The listing builds one solid part. Answer for the finished solid, in the listing's coordinates (mm). A direction names the side the tool comes from. Round coordinates to 2 decimals unless told otherwise and drop trailing zeros. Write each loop counter-clockwise with the first axis right and the second up, starting at its lowest first coordinate (ties: lowest second). Pieces come first, ordered by that corner, then holes. Notation, with made-up numbers: (-10.5, 21.5) - (-6.5, 21.5) arc R19 cw to (-6.5, 36.5) - close; hole circle Ø1 at (10, 88.25). An arc over 180 degrees is marked (long way). Answer as CSV lines item,"result". Start each with the question number.
Item 1: A cutting plane is placed at B-B on x = 0. Determine the outline of the cut face in (y, z), and give its area (3 significant figures).
Item 2: Straight lines are drawn through the part: line 1 along Z through (x, y) = (-1.5, 2.25); line 2 along Z through (x, y) = (-1.25, 5.25); line 3 along Y through (x, z) = (-2.25, 1.5). For each, find the intervals that lie inside material, in ascending order. Write a range as [from, to].
Item 3: Which of the six approach directions +Z, -Z, +X, -X, +Y, -Y give full straight-line access (tool end or side, diameter ignored) to faces 1 (the cylindrical face through (-0.54, 1.48, -2.44)), 2 (the flat face through (0, 0, 0))?
Item 4: Flat-ended cylindrical pins translate along their axes: pin 1 (4 mm diameter, centred on y = 1.5, z = -1.5, fed in from -X); pin 2 (3 mm diameter, centred on x = -2, y = 2.5, fed in from +Z); pin 3 (2 mm diameter, centred on y = 5.5, z = -0.5, fed in from -X). Find the tip coordinate at first contact, or state that the pin passes through.
Item 5: A cutting plane is placed at C-C on y = 2.75. Determine the outline of the cut face in (x, z), and give its area (3 significant figures).
Item 6: A cutting plane is placed at A-A on z = 0. Determine the outline of the cut face in (x, y), and give its area (3 significant figures).
Item 7: A cutting plane is placed at D-D on y = 3.5. Determine the outline of the cut face in (x, z).
Autodesk Inventor part; units mm, degrees
ref_plane "YZ Plane" through (0, 0, 0) normal (1, 0, 0) x (0, 1, 0)
ref_plane "XZ Plane" through (0, 0, 0) normal (0, 1, 0) x (-1, 0, 0)
ref_plane "XY Plane" through (0, 0, 0) normal (0, 0, 1) x (1, 0, 0)
sketch "Szkic1" plane through (0, 0, 0) normal (0, 1, 0) x (-1, 0, 0)
  circle A0 centre (0, 0) radius 4
  dimension "d0" = 8
extrude "Wyciągnięcie proste1" add sketch "Szkic1" along normal blind 7
fillet "Zaokrąglenie1" radius 4 1 edges at (4, 7, 0)
sketch "Szkic2" plane through (0, 0, 0) normal (0, -1, 0) x (1, 0, 0)
  circle A0 centre (0, 0) radius 2.5
  circle A1 centre (0, 0) radius 4
  dimension "d4" = 5
  dimension "d5" = 8
extrude "Wyciągnięcie proste2" cut sketch "Szkic2" against normal blind 3
properties part number "GumoweTrzymadlo" material "Tworzywo sztuczne PET"
Geometry says:
1,outline,"(0, -2.5) - (3, -2.5) - (3, -4) arc R4 ccw to (3, 4) - (3, 2.5) - (0, 2.5) - close"
1,area,"40.1 mm^2"
2,line 1,"z = [-2, 2]"
2,line 2,"z = [-3.06, 3.06]"
2,line 3,"y = [3, 5.95]"
3,face 1,"-Y"
3,face 2,"+Z, -Z, +X, -X, -Y"
4,pin 1,"stops at x = -4"
4,pin 2,"stops at z = 3.96"
4,pin 3,"stops at x = -3.69"
5,outline,"circle Ø5 at (0, 0)"
5,area,"19.6 mm^2"
6,outline,"(-4, 3) - (-2.5, 3) - (-2.5, 0) - (2.5, 0) - (2.5, 3) - (4, 3) arc R4 ccw to start"
6,area,"40.1 mm^2"
7,outline,"circle Ø7.94 at (0, 0)"
